Could you check a few things on this model? Use its own coordinates, in mm. A direction names the side the tool comes from. Round coordinates to 2 decimals unless told otherwise and drop trailing zeros. Write each loop counter-clockwise with the first axis right and the second up, starting at its lowest first coordinate (ties: lowest second). Pieces come first, ordered by that corner, then holes. Notation, with made-up numbers: (77.5, 31.25) - (134.5, 31.25) arc R19 cw to (134.5, 50.25) - close; hole circle Ø1 at (82.25, -23.5). An arc over 180 degrees is marked (long way). Write each question's results on one line, items separated by ' | '. Start each with the question number.
(1) Thinking about a two-plate mould opening in X: for faces 1 (the cylindrical face through (1.32, -2.46, 29.97)), 2 (the flat face through (25, 0, 7)), 3 (the cylindrical face through (-10.885, 6.902, -2.417)), which applies, +X half, -X half, draft (parallel to the pull), parting line (faces both ways), or undercut?
(2) Imagine slicing it at A-A on x = 0. Write out the boundary of the cut face in (y, z), then the cut area to 3 significant figures.
(3) Imagine slicing it at D-D on y = 12.25. Write out the boundary of the cut face in (x, z).
(4) Imagine slicing it at B-B on z = 0. Write out the boundary of the cut face in (x, y).
(5) Please list where these lines run through material, in increasing order: line 1 (X direction, y = 6.5, z = 0); line 2 (X direction, y = 9, z = 0); line 3 (Y direction, x = -18.5, z = -8). Write a range as [from, to].
(6) For P1, Ø1, axis at y = 4, z = 9, coming from the -X side; P2, Ø1.5, axis at y = 7.5, z = -11, coming from the +X side; P3, Ø10, axis at y = -2, z = -11.5, coming from the -X side, each with a flat end and sliding along its axis, tell me the tip position at first contact or that it passes through.
(7) Imagine slicing it at C-C on z = -24. Write out the boundary of the cut face in (x, y).
(8) On a 3-axis mill with a long thin cutter (end or side, diameter ignored), from which of +Z, -Z, +X, -X, +Y, -Y can I reach the whole of each face in a straight line? I mean faces 4 (the flat face through (-20, -5, -6)), 5 (the cylindrical face through (-5.42, 10.45, 13.07)), 6 (the flat face through (-9, 0, 9)). Say none if no direction works.
```python
from build123d import *

# Parameters (mm, degrees)
SKETCH1_R           = 25
SKETCH1_R_2         = 11.15
BOSS_EXTRUDE1_DEPTH = 7
SKETCH2_R           = 14.15
SKETCH2_R_2         = 11.15
BOSS_EXTRUDE2_DEPTH = 7
SKETCH3_R           = 30
SKETCH3_R_2         = 20
BOSS_EXTRUDE3_DEPTH = 5


with BuildPart() as part:
    # Sketch1 → Boss-Extrude1 (new body)
    with BuildSketch(Plane(origin=(0, 0, 0), x_dir=(1, 0, 0), z_dir=(0, 1, 0))):
        with Locations(Location((0, 0, 0), (0, 0, 270))):
            Circle(SKETCH1_R)
        with Locations(Location((0, 0, 0), (0, 0, 270))):
            Circle(SKETCH1_R_2, mode=Mode.SUBTRACT)
    extrude(amount=BOSS_EXTRUDE1_DEPTH)

    # Sketch2 → Boss-Extrude2 (add)
    with BuildSketch(Plane(origin=(0, 7, 0), x_dir=(1, 0, 0), z_dir=(0, 1, 0))):
        with Locations(Location((0, 0, 0), (0, 0, 270))):
            Circle(SKETCH2_R)
        with Locations(Location((0, 0, 0), (0, 0, 270))):
            Circle(SKETCH2_R_2, mode=Mode.SUBTRACT)
    extrude(amount=BOSS_EXTRUDE2_DEPTH)

    # Sketch3 → Boss-Extrude3 (add)
    with BuildSketch(Plane.XZ):
        with Locations(Location((0, 0, 0), (0, 0, 270))):
            Circle(SKETCH3_R)
        with Locations(Location((0, 0, 0), (0, 0, 270))):
            Circle(SKETCH3_R_2, mode=Mode.SUBTRACT)
    extrude(amount=BOSS_EXTRUDE3_DEPTH)


solid = part.part
```
Response:
1) face 1: parting line | face 2: draft | face 3: undercut
2) outline: (-5, -30) - (0, -30) - (0, -25) - (7, -25) - (7, -14.15) - (14, -14.15) - (14, -11.15) - (0, -11.15) - (0, -20) - (-5, -20) - close; (-5, 20) - (0, 20) - (0, 11.15) - (14, 11.15) - (14, 14.15) - (7, 14.15) - (7, 25) - (0, 25) - (0, 30) - (-5, 30) - close | area: 336 mm²
3) outline: circle Ø28.3 at (0, 0); hole circle Ø22.3 at (0, 0)
4) outline: (-30, -5) - (-20, -5) - (-20, 0) - (-11.15, 0) - (-11.15, 14) - (-14.15, 14) - (-14.15, 7) - (-25, 7) - (-25, 0) - (-30, 0) - close; (11.15, 0) - (20, 0) - (20, -5) - (30, -5) - (30, 0) - (25, 0) - (25, 7) - (14.15, 7) - (14.15, 14) - (11.15, 14) - close
5) line 1: [-25, -11.15], [11.15, 25] | line 2: [-14.15, -11.15], [11.15, 14.15] | line 3: [-5, 7]
6) P1: x = -23.51 | P2: x = 22.72 | P3: x = -29.29
7) outline: (-18, -5) - (18, -5) - (18, 0) - (7, 0) - (7, 7) - (-7, 7) - (-7, 0) - (-18, 0) - close
8) face 4: +Z, -Z, +X, -X, -Y | face 5: +Y | face 6: -Y
